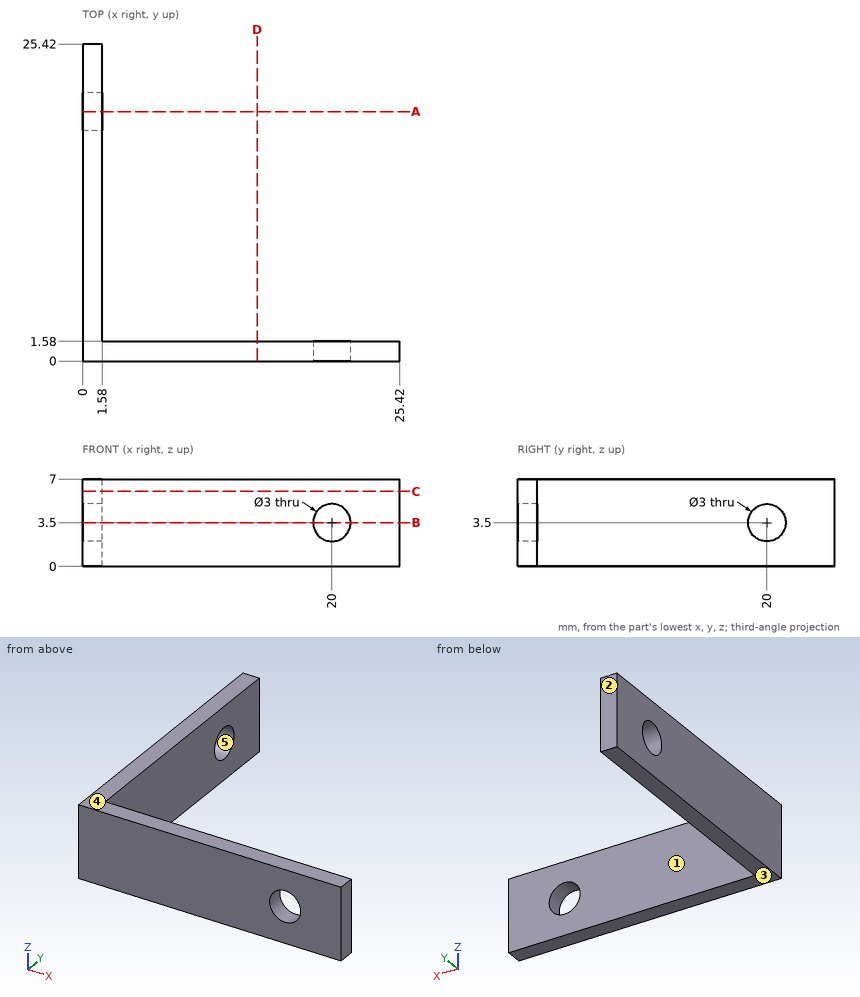
Design review of the part shown in the three views and the two pictorial views. Dimensions are in mm from the part's minimum x, y and z. A direction names the side the tool comes from. Round coordinates to 2 decimals unless told otherwise and drop trailing zeros. Write each loop counter-clockwise with the first axis right and the second up, starting at its lowest first coordinate (ties: lowest second). Pieces come first, ordered by that corner, then holes. Notation, with made-up numbers: M 81,26.5 L 137,26.5 A9 cw 137,34.5 Z; hole C -9,0 d5. An arc over 180 degrees is marked long. Use a Markdown table: item, result. Add a question column.
Q1. The part is to be moulded in two halves that separate along Z. For the marked faces 3, 4 and 5, say which applies: pulls with the +Z half, pulls with the -Z half, needs draft (parallel to the pull), parting line crosses it, or undercut.
Q2. To check wall thickness, follow line 1 (Z direction, x = 20, y = 0.45); line 2 (X direction, y = 15, z = 1.25). State the ranges of each line that lie inside material, in increasing order.
Q3. We need section B-B, the plane z = 3.5. State the section outline as (x, y) points.
Q4. We need section D-D, the plane x = 14. State the section outline as (y, z) points, plus the area to 3 significant figures.
Q5. Insertion check: pin 1 (3.5 mm diameter, centred on x = 12.5, z = 3, fed in from +Y); pin 2 (2 mm diameter, centred on y = 13, z = 4, fed in from +X); pin 3 (10 mm diameter, centred on x = 19, y = 10, fed in from +Z). Each pin has a flat end and moves straight along its axis. Give the tip position at first contact, or say it passes through.
Q6. Machinability: for the marked faces 1 and 2, which of the approach directions +Z, -Z, +X, -X, +Y, -Y give a long, thin tool a straight path to every point of the face, cutting with its end or side? Answer none if there is none.
Q7. We need section A-A, the plane y = 20. State the section outline as (x, z) points, plus the area to 3 significant figures.
Q8. We need section C-C, the plane z = 6. State the section outline as (x, y) points, plus the area to 3 significant figures.
Findings below:
| question | item | result |
|---|---|---|
| 1 | face 3 | pulls with the -Z half |
| 1 | face 4 | pulls with the +Z half |
| 1 | face 5 | undercut |
| 2 | line 1 | z = 0 to 2, 5 to 7 |
| 2 | line 2 | x = 0 to 1.58 |
| 3 | outline | M 0,0 L 18.5,0 L 18.5,1.58 L 1.58,1.58 L 1.58,18.5 L 0,18.5 Z; M 0,21.5 L 1.58,21.5 L 1.58,25.42 L 0,25.42 Z; M 21.5,0 L 25.42,0 L 25.42,1.58 L 21.5,1.58 Z |
| 4 | outline | M 0,0 L 1.58,0 L 1.58,7 L 0,7 Z |
| 4 | area | 11.1 mm² |
| 5 | pin 1 | stops at y = 1.58 |
| 5 | pin 2 | stops at x = 1.58 |
| 5 | pin 3 | passes through |
| 6 | face 1 | +Z, -Z, +X, +Y |
| 6 | face 2 | +Z, -Z, +X, -X, +Y |
| 7 | outline | M 0,0 L 1.58,0 L 1.58,2 L 0,2 Z; M 0,5 L 1.58,5 L 1.58,7 L 0,7 Z |
| 7 | area | 6.32 mm² |
| 8 | outline | M 0,0 L 25.42,0 L 25.42,1.58 L 1.58,1.58 L 1.58,25.42 L 0,25.42 Z |
| 8 | area | 77.8 mm² |
